```python
from build123d import *

# Parameters (mm, degrees)
PAD011_DEPTH    = 12
POCKET009_DEPTH = 11.401
POCKET010_DEPTH = 5


with BuildPart() as part:
    # Sketch031 → Pad011 (new body)
    with BuildSketch(Plane.XY):
        with BuildLine():
            ThreePointArc((16.4829457319, -0.75), (7.6571484981, 14.6156791453), (-10, 13.1244047484))
            Line((-10, 8.85), (-10, 13.1244047484))
            Line((-2.5, 8.85), (-10, 8.85))
            Line((-2.5, 0.75), (-2.5, 8.85))
            Line((-16.4829457319, 0.75), (-2.5, 0.75))
            ThreePointArc((-16.4829457319, 0.75), (-7.6571484981, -14.6156791453), (10, -13.1244047484))
            Line((10, -13.1244047484), (10, -8.85))
            Line((10, -8.85), (2.5, -8.85))
            Line((2.5, -8.85), (2.5, -0.75))
            Line((16.4829457319, -0.75), (2.5, -0.75))
        make_face()
    extrude(amount=-PAD011_DEPTH)

    # Sketch032 → Pocket009 (cut, through all)
    with BuildSketch(Plane.XY.offset(-0.6)):
        Polygon((-0.55, 3.043445), (9.55, 3.043445), (9.55, 1.943445), (0.55, 1.943445), (0.55, -7.056555), (-0.55, -7.056555), align=None)
    extrude(amount=-POCKET009_DEPTH, mode=Mode.SUBTRACT)

    # Sketch035 → Pocket010 (cut)
    with BuildSketch(Plane.XY.offset(-10)):
        Polygon((0.55, 2.15), (1.65, 2.15), (1.65, -8.15), (-8.45, -8.15), (-8.45, -7.05), (0.55, -7.05), align=None)
    extrude(amount=-POCKET010_DEPTH, mode=Mode.SUBTRACT)

    # Sketch046 → Groove (revolve, cut)
    with BuildSketch(Plane.YZ):
        Polygon((16.5, 0), (16.5, -1.080549), (14.935277, -1.996929), (14.625, -13.52658), (22.461165, -13.52658), (22.461165, 0), align=None)
    revolve(axis=Axis((0, 0, 0), (0, 0, 1)), mode=Mode.SUBTRACT)


solid = part.part
```
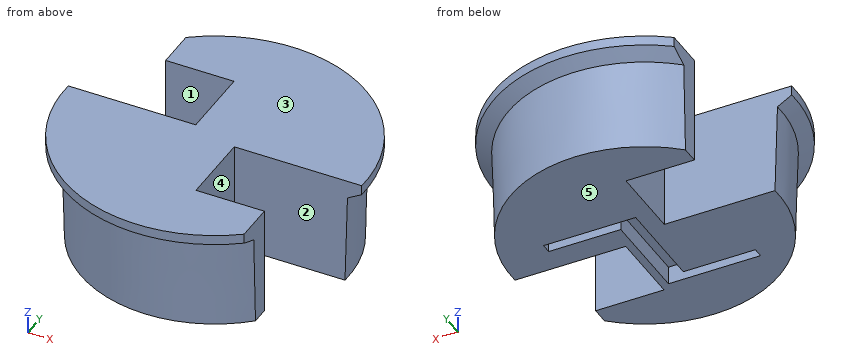
Here's how the part is built. I have some questions about the finished solid (model axes, mm). Face numbers are marked on the shaded views. A direction names the side the tool comes from. Coordinates: 2 decimals unless noted, no trailing zeros. Write each loop counter-clockwise with the first axis right and the second up, starting at its lowest first coordinate (ties: lowest second). Pieces come first, ordered by that corner, then holes. Notation, with made-up numbers: (27, 62.5) -> (60, 62.5) arc R23 cw to (60, 78.5) -> close; hole circle Ø9 at (87, -0.75). An arc over 180 degrees is marked (long way). Use a Markdown table: item, result. Add a question column.
(1) I'm going to push flat-ended pins straight in: P1, Ø2.5, axis at y = -4, z = -7.5, coming from the -X side; P2, Ø4, axis at x = 5, z = -3.5, coming from the +Y side; P3, Ø4, axis at x = -4.5, z = -7, coming from the -Y side; P4, Ø4, axis at x = 6.5, y = 1, coming from the +Z side. Where does each tip first touch, or does it pass through?
(2) If we section it at C-C, the plane y = 0: Write out the boundary of the cut face in (x, z).
(3) If we section it at D-D, the plane z = -7.75: Write out the boundary of the cut face in (x, y).
(4) For the marked faces 1, 2 and 3, which set-ups out of +Z, -Z, +X, -X, +Y, -Y let a thin tool reach every point of the face, with its end or its side?
(5) If we section it at B-B, the plane x = 0: Write out the boundary of the cut face in (y, z).
(6) If we section it at A-A, the plane z = -2.5: Write out the boundary of the cut face in (x, y), and give its area (3 significant figures).
(7) We'd pull the mould along Y, two halves only. Please class the marked faces 4 and 5: +Y half, -Y half, draft (parallel to the pull), parting line (faces both ways), or undercut.
(8) Please list where these lines run through material, in increasing order: line 1 (Y direction, x = 4, z = -1.25); line 2 (Y direction, x = 5.5, z = -8.5); line 3 (X direction, y = -0.5, z = -8.75).
Outcome:
| question | item | result |
|---|---|---|
| 1 | P1 | stops at x = -14.53 |
| 1 | P2 | stops at y = 15.03 |
| 1 | P3 | stops at y = -14.59 |
| 1 | P4 | stops at z = 0 |
| 2 | outline | (-16.5, -1.08) -> (-14.94, -2) -> (-14.67, -12) -> (-0.55, -12) -> (-0.55, -0.6) -> (0.55, -0.6) -> (0.55, -10) -> (1.65, -10) -> (1.65, -12) -> (14.67, -12) -> (14.94, -2) -> (16.5, -1.08) -> (16.5, 0) -> (-16.5, 0) -> close |
| 3 | outline | (-14.76, 0.75) arc R14.78 ccw to (10, -10.88) -> (10, -8.85) -> (2.5, -8.85) -> (2.5, -0.75) -> (14.76, -0.75) arc R14.78 ccw to (-10, 10.88) -> (-10, 8.85) -> (-2.5, 8.85) -> (-2.5, 0.75) -> close; hole (-0.55, -7.06) -> (0.55, -7.06) -> (0.55, 1.94) -> (9.55, 1.94) -> (9.55, 3.04) -> (-0.55, 3.04) -> close |
| 4 | face 1 | +Z, -Z, -X |
| 4 | face 2 | +Z, -Z, +X |
| 4 | face 3 | +Z, +X, -X, +Y, -Y |
| 5 | outline | (-16.5, -1.08) -> (-14.94, -2) -> (-14.67, -12) -> (-8.15, -12) -> (-8.15, -10) -> (-7.06, -10) -> (-7.06, -0.6) -> (3.04, -0.6) -> (3.04, -12) -> (14.67, -12) -> (14.94, -2) -> (16.5, -1.08) -> (16.5, 0) -> (-16.5, 0) -> close |
| 6 | outline | (-14.9, 0.75) arc R14.92 ccw to (10, -11.08) -> (10, -8.85) -> (2.5, -8.85) -> (2.5, -0.75) -> (14.9, -0.75) arc R14.92 ccw to (-10, 11.08) -> (-10, 8.85) -> (-2.5, 8.85) -> (-2.5, 0.75) -> close; hole (-0.55, -7.06) -> (0.55, -7.06) -> (0.55, 1.94) -> (9.55, 1.94) -> (9.55, 3.04) -> (-0.55, 3.04) -> close |
| 6 | area | 489 mm^2 |
| 7 | face 4 | undercut |
| 7 | face 5 | draft |
| 8 | line 1 | y = -15.71 to -8.85, -0.75 to 1.94, 3.04 to 15.71 |
| 8 | line 2 | y = -13.7 to -8.85, -0.75 to 1.94, 3.04 to 13.7 |
| 8 | line 3 | x = -14.75 to -0.55, 0.55 to 14.75 |
